```python
from build123d import *

# Parameters (mm, degrees)
F1_DEPTH  = 12.7
F3_DEPTH  = 7.85
F4_W      = 59.69
F4_H      = 9.652
F5_DEPTH  = 127.001
F6_W      = 76.2
F6_H      = 50.8
F7_DEPTH  = 5.08
F9_W      = 62.4130927026
F9_H      = 11.1426808871
F10_DEPTH = 0.254


with BuildPart() as f1:
    # F0 (on Top) → F1 (new body, symmetric)
    with BuildSketch(Plane.XY):
        with BuildLine():
            ThreePointArc((-10.3697649443, -3), (0, 10.795), (10.3697649443, -3))
            Line((10.3697649443, -3), (13.4648440392, -3))
            ThreePointArc((13.4648440392, -3), (13.7122125954, -1.5090562414), (13.795, 0))
            ThreePointArc((13.795, 0), (0, 13.795), (-13.795, 0))
            ThreePointArc((-13.795, 0), (-13.7122125954, -1.5090562414), (-13.4648440392, -3))
            Line((-13.4648440392, -3), (-10.3697649443, -3))
        make_face()
    extrude(amount=F1_DEPTH, both=True)

    # F2 (on Top) → F3 (join, symmetric)
    with BuildSketch(Plane.XY):
        with BuildLine():
            Line((63.5, 13.794994), (63.5, 83.644994))
            Line((63.5, 83.644994), (-63.5, 83.644994))
            Line((-63.5, 83.644994), (-63.5, 13.794994))
            Line((-63.5, 13.794994), (-13.794994, 0))
            ThreePointArc((-13.794994, 0), (0, 13.794994), (13.794994, 0))
            Line((13.794994, 0), (63.5, 13.794994))
        make_face()
    extrude(amount=F3_DEPTH, both=True)

    # F4 (on face) → F5 (cut, through all)
    with BuildSketch(Plane.YZ.offset(63.5)):
        with Locations((48.719994, -0.1927575009)):
            Rectangle(F4_W, F4_H)
    extrude(amount=-F5_DEPTH, mode=Mode.SUBTRACT)

    # F6 (on face) → F7 (cut)
    with BuildSketch(Plane.XY.offset(7.85)):
        with Locations((0, 48.719994)):
            Rectangle(F6_W, F6_H)
    extrude(amount=-F7_DEPTH, mode=Mode.SUBTRACT)

    # F9 (on face) → F10 (join)
    with BuildSketch(Plane(origin=(-63.5, 0, 0), x_dir=(0, -1, 0), z_dir=(-1, 0, 0))):
        with Locations((-48.8958675414, -0.0143751968)):
            Rectangle(F9_W, F9_H)
    extrude(amount=-F10_DEPTH)


solid = f1.part
```
For this review, take the finished solid that the model builds, in its own axes (mm). A direction names the side the tool comes from. Round coordinates to 2 decimals unless told otherwise and drop trailing zeros. Loops run counter-clockwise (first coordinate to the right, second up) from the corner with the lowest first, then second, coordinate; pieces in that order, holes last.
Q1. Add section D-D on x = 0. Write out the cut boundary in (y, z) (3 decimals).
Result sheet:
outline: (10.795, -12.7) - (13.795, -12.7) - (13.795, -7.85) - (83.645, -7.85) - (83.645, 7.85) - (74.12, 7.85) - (74.12, 4.633) - (78.565, 4.633) - (78.565, -5.019) - (18.875, -5.019) - (18.875, 4.633) - (23.32, 4.633) - (23.32, 7.85) - (13.795, 7.85) - (13.795, 12.7) - (10.795, 12.7) - close
Q2. Add section A-A on y = 63. Write out the cut boundary in (x, z), plus the area to 3 significant figures.
Result sheet:
outline: (-63.5, -7.85) - (63.5, -7.85) - (63.5, -5.02) - (-63.25, -5.02) - (-63.25, 4.63) - (-38.1, 4.63) - (-38.1, 7.85) - (-63.5, 7.85) - close; (38.1, 4.63) - (63.5, 4.63) - (63.5, 7.85) - (38.1, 7.85) - close
area: 525 mm2
Q3. Mouldability with a two-part tool opening along X and no side actions: class faces 6 (the face through (2, 11, -12.7)), 7 (the face through (63.5, 48, 5)), 8 (the face through (-0.28, 10.79, 0.18)) as +X half, -X half, draft (parallel to the pull), parting line (faces both ways), or undercut.
Result sheet:
face 6: draft
face 7: +X half
face 8: undercut
Q4. Add section B-B on x = -43.5. Write out the cut boundary in (y, z) (3 decimals).
Result sheet:
outline: (8.244, -7.85) - (83.645, -7.85) - (83.645, 7.85) - (8.244, 7.85) - close; hole (18.875, -5.019) - (78.565, -5.019) - (78.565, 4.633) - (18.875, 4.633) - close
Q5. Insertion check: pin 1 Ø25 at (x, y) = (21.5, 50) entering from +Z; pin 2 Ø10.5 at (x, z) = (-4, -1.5) entering from -Y (3 decimals); pin 3 Ø5 at (y, z) = (59.5, -2) entering from +X. Each pin has a flat end and moves straight along its axis. Give the tip position at first contact, or say it passes through.
Result sheet:
pin 1: stops at z = -5.02
pin 2: stops at y = 5.565
pin 3: stops at x = -63.25
Q6. To check wall thickness, follow line 1 along Y through (x, z) = (0, 1.75) (3 decimals); line 2 along Z through (x, y) = (45.5, 75); line 3 along Z through (x, y) = (17.5, 10). State the ranges of each line that lie inside material, in increasing order.
Result sheet:
line 1: y = 10.795 to 18.875, 78.565 to 83.645
line 2: z = -7.85 to -5.02, 4.63 to 7.85
line 3: z = -7.85 to 7.85
Q7. Machinability: for faces 1 (the face through (-38.995, 6.994, 0.11)), 2 (the face through (-38.1, 48, 6)), 3 (the face through (5.66, 12.58, 8.64)), 4 (the face through (1, 18.875, 0)), 5 (the face through (1, 83.645, 0)), which of the approach directions +Z, -Z, +X, -X, +Y, -Y give a long, thin tool a straight path to every point of the face, cutting with its end or side? Answer none if there is none.
Result sheet:
face 1: +Z, -Z, -X, -Y
face 2: +Z
face 3: none
face 4: +X
face 5: +Z, -Z, +X, -X, +Y
Q8. Add section C-C on z = 0.75. Write out the cut boundary in (x, y) (3 decimals), plus the area to 3 significant figures.
Result sheet:
outline: (-63.5, 13.795) - (-13.795, 0) arc R13.795 ccw to (-13.465, -3) - (-10.37, -3) arc R10.795 cw (long way) to (10.37, -3) - (13.465, -3) arc R13.795 ccw to (13.795, 0) - (63.5, 13.795) - (63.5, 18.875) - (-63.246, 18.875) - (-63.246, 78.565) - (63.5, 78.565) - (63.5, 83.645) - (-63.5, 83.645) - close
area: 2,210 mm2
